Can you work these out from the drawing? Everything is in mm from the part's minimum corner. A direction names the side the tool comes from. Round coordinates to 2 decimals unless told otherwise and drop trailing zeros. Write each loop counter-clockwise with the first axis right and the second up, starting at its lowest first coordinate (ties: lowest second). Pieces come first, ordered by that corner, then holes. Notation, with made-up numbers: (-15.5, -12.5) -> (29.5, -12.5) arc R12 cw to (29.5, -4.5) -> close; hole circle Ø8 at (72.25, 24.25). An arc over 180 degrees is marked (long way). One line per question, with ' | ' between items. Start each with the question number.
1. Imagine slicing it at C-C, the plane x = 5.5. List the corners of the cut face in (y, z) for me, and give its area (3 significant figures).
2. Imagine slicing it at B-B, the plane x = 21.5. List the corners of the cut face in (y, z) for me.
3. Imagine slicing it at A-A, the plane z = 21.5. List the corners of the cut face in (x, y) for me.
4. Thinking about a two-plate mould opening in Z: for the marked faces 3, 4, 5 and 6, which applies, released by +Z, released by -Z, zero draft, split by the parting line, or undercut?
5. If I drill on line 1 along X through (y, z) = (42.9, 3.5); line 2 along X through (y, z) = (43, 18); line 3 along X through (y, z) = (43, 10.75), over which ranges is the centre line in solid material (lowest first)? Write a range as [from, to].
6. For the marked faces 1 and 2, which set-ups out of +Z, -Z, +X, -X, +Y, -Y let a thin tool reach every point of the face, with its end or its side?
7. Imagine slicing it at D-D, the plane y = 33.5. List the corners of the cut face in (x, z) for me.
8. For pin 1 Ø3 at (x, z) = (9, 19.5) entering from -Y; pin 2 Ø2.5 at (y, z) = (22, 10.5) entering from +X; pin 3 Ø1.6 at (y, z) = (1, 13) entering from -X, each with a flat end and sliding along its axis, tell me the tip position at first contact or that it passes through.
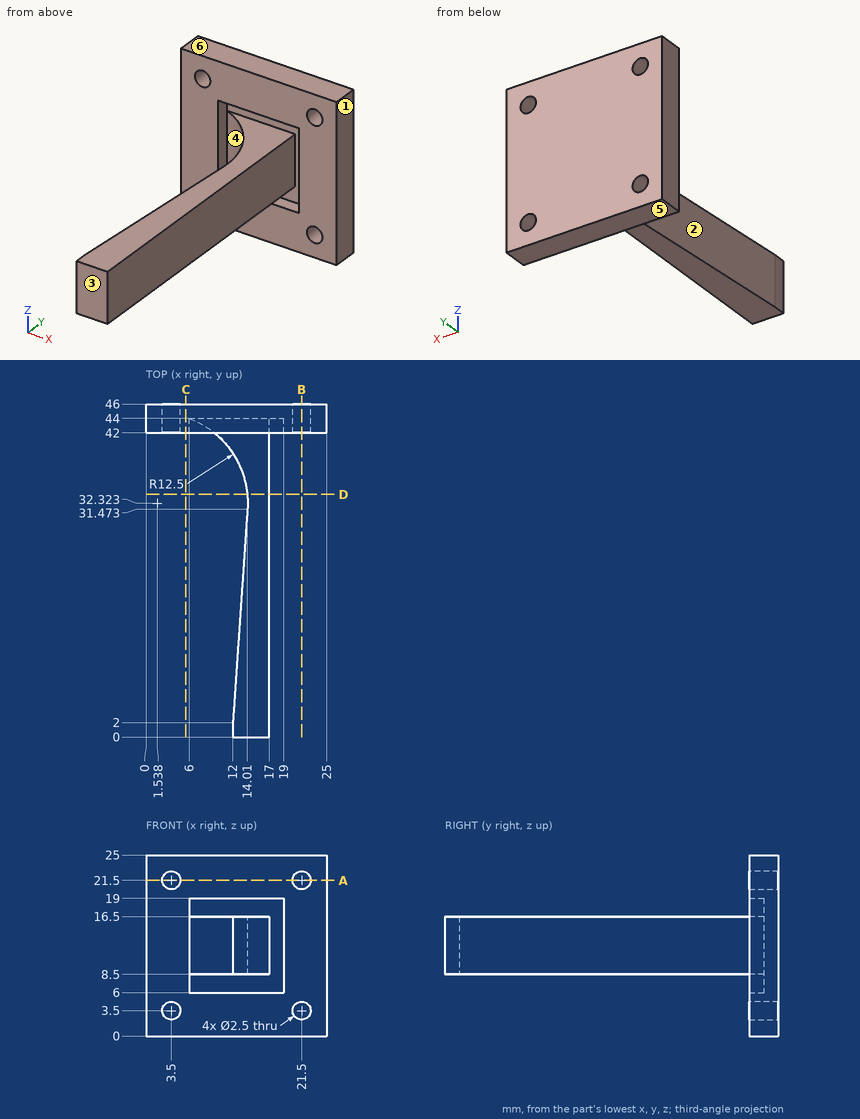
Geometry results:
1) outline: (42, 0) -> (46, 0) -> (46, 25) -> (42, 25) -> close | area: 100 mm2
2) outline: (42, 0) -> (46, 0) -> (46, 2.25) -> (42, 2.25) -> close; (42, 4.75) -> (46, 4.75) -> (46, 20.25) -> (42, 20.25) -> close; (42, 22.75) -> (46, 22.75) -> (46, 25) -> (42, 25) -> close
3) outline: (0, 42) -> (2.25, 42) -> (2.25, 46) -> (0, 46) -> close; (4.75, 42) -> (20.25, 42) -> (20.25, 46) -> (4.75, 46) -> close; (22.75, 42) -> (25, 42) -> (25, 46) -> (22.75, 46) -> close
4) face 3: zero draft | face 4: undercut | face 5: released by -Z | face 6: released by +Z
5) line 1: x = [0, 2.25], [4.75, 20.25], [22.75, 25] | line 2: x = [0, 6], [19, 25] | line 3: x = [0, 6], [8.04, 17], [19, 25]
6) face 1: +Z, -Z, +X, +Y, -Y | face 2: +Z, -Z, -X
7) outline: (13.98, 8.5) -> (17, 8.5) -> (17, 16.5) -> (13.98, 16.5) -> close
8) pin 1: stops at y = 42 | pin 2: stops at x = 17 | pin 3: stops at x = 12
